Design review of the part built by this model. Coordinates are the model's own, in mm. Face numbers are marked on the shaded views. A direction names the side the tool comes from. Round coordinates to 2 decimals unless told otherwise and drop trailing zeros. Order: outer loops, then holes, each group sorted by start corner. A loop starts at its lowest first (then second) coordinate and runs counter-clockwise, first axis right, second up. Notation, with made-up numbers: (27.5, 29.25) - (59.5, 29.25) arc R20 cw to (59.5, 43.25) - close; hole circle Ø7 at (62, 16.5). An arc over 180 degrees is marked (long way). Write item = value, one per line.
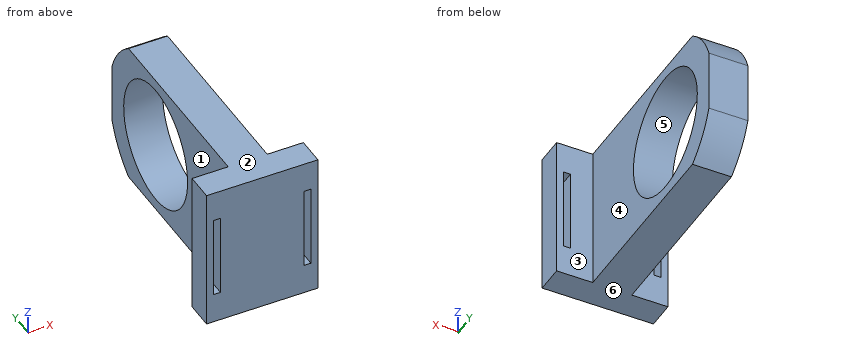
from build123d import *

# Parameters (mm, degrees)
SKETCH1_W           = 20
SKETCH1_H           = 26
SKETCH1_W_2         = 1.25
SKETCH1_H_2         = 15
BOSS_EXTRUDE5_DEPTH = 5
SKETCH3_W           = 7
SKETCH3_H           = 26
BOSS_EXTRUDE6_DEPTH = 40
CUT_EXTRUDE1_REACH  = 55.696
SKETCH5_R           = 11


with BuildPart() as part:
    # Sketch1 → Boss-Extrude5 (new body)
    with BuildSketch(Plane(origin=(0, 0, 0), x_dir=(1, 0, 0), z_dir=(0, 1, 0))):
        with Locations((10, 13)):
            Rectangle(SKETCH1_W, SKETCH1_H)
        with Locations((1.875, 13)):
            Rectangle(SKETCH1_W_2, SKETCH1_H_2, mode=Mode.SUBTRACT)
        with Locations((18.125784532, 13)):
            Rectangle(SKETCH1_W_2, SKETCH1_H_2, mode=Mode.SUBTRACT)
    extrude(amount=BOSS_EXTRUDE5_DEPTH)

    # Sketch3 → Boss-Extrude6 (add)
    with BuildSketch(Plane(origin=(0, 5, 0), x_dir=(1, 0, 0), z_dir=(0, 1, 0))):
        with Locations((10, 13)):
            Rectangle(SKETCH3_W, SKETCH3_H)
    extrude(amount=BOSS_EXTRUDE6_DEPTH)

    # Sketch5 → Cut-Extrude1 (cut, up to next)
    with BuildSketch(Plane(origin=(13.5, 0, 0), x_dir=(0, 0, -1), z_dir=(1, 0, 0)), mode=Mode.PRIVATE) as cut_extrude1_sk1:
        with Locations((13, 30)):
            Circle(SKETCH5_R)
    cut_extrude1_tool1 = extrude(cut_extrude1_sk1.sketch, amount=-CUT_EXTRUDE1_REACH, mode=Mode.PRIVATE) & part.part
    # Sketch5 → Cut-Extrude1 (cut, up to next)
    with BuildSketch(Plane(origin=(13.5, 0, 0), x_dir=(0, 0, -1), z_dir=(1, 0, 0)), mode=Mode.PRIVATE) as cut_extrude1_sk2:
        with BuildLine():
            Line((7.432235637, 45), (0, 45))
            Line((0, 45), (0, 39.327379053))
            ThreePointArc((0, 39.327379053), (3.292522189, 42.718682107), (7.432235637, 45))
        make_face()
    cut_extrude1_tool2 = extrude(cut_extrude1_sk2.sketch, amount=-CUT_EXTRUDE1_REACH, mode=Mode.PRIVATE) & part.part
    # Sketch5 → Cut-Extrude1 (cut, up to next)
    with BuildSketch(Plane(origin=(13.5, 0, 0), x_dir=(0, 0, -1), z_dir=(1, 0, 0)), mode=Mode.PRIVATE) as cut_extrude1_sk3:
        with BuildLine():
            Line((26, 39.327379053), (26, 45))
            Line((26, 45), (18.567764363, 45))
            ThreePointArc((18.567764363, 45), (22.707477811, 42.718682107), (26, 39.327379053))
        make_face()
    cut_extrude1_tool3 = extrude(cut_extrude1_sk3.sketch, amount=-CUT_EXTRUDE1_REACH, mode=Mode.PRIVATE) & part.part
    add(cut_extrude1_tool1.solids().sort_by_distance((13.5, 30, -13))[0], mode=Mode.SUBTRACT)
    add(cut_extrude1_tool2.solids().sort_by_distance((13.5, 43.298273, -2.197768))[0], mode=Mode.SUBTRACT)
    add(cut_extrude1_tool3.solids().sort_by_distance((13.5, 43.298273, -23.802232))[0], mode=Mode.SUBTRACT)


solid = part.part
1) We need section C-C on z = -13. Write out the cut boundary in (x, y), and give its area (4 significant figures).
Findings:
outline = (0, 0) - (1.25, 0) - (1.25, 5) - (0, 5) - close; (2.5, 0) - (17.5, 0) - (17.5, 5) - (13.5, 5) - (13.5, 19) - (6.5, 19) - (6.5, 5) - (2.5, 5) - close; (6.5, 41) - (13.5, 41) - (13.5, 45) - (6.5, 45) - close; (18.75, 0) - (20, 0) - (20, 5) - (18.75, 5) - close
area = 213.5 mm^2
2) To check wall thickness, follow L1, parallel to Y at x = 8, z = -13; L2, parallel to X at y = 39, z = -4; L3, parallel to Y at x = 17, z = -14.5. State the ranges of each line that lie inside material, in increasing order. Write a range as from..to.
Findings:
L1 = 0..19, 41..45
L2 = 6.5..13.5
L3 = 0..5
3) Clearance check with flat-ended pins moving along their axes: pin 1 Ø2 at (x, z) = (16.5, -13) entering from +Y; pin 2 Ø6 at (y, z) = (9, -5.5) entering from -X; pin 3 Ø2 at (x, y) = (15.5, 35.5) entering from -Z. State where each tip first meets the part, or that it passes through.
Findings:
pin_1 = 5
pin_2 = 6.5
pin_3 = through
4) For the marked faces 1, 2 and 3, list the 3-axis set-ups (+Z, -Z, +X, -X, +Y, -Y) from which the entire face can be reached by the end or side of a thin tool; tool diameter is ignored.
Findings:
face_1 = +Z, -Z, -X, +Y
face_2 = +Z, +X, -X, +Y, -Y
face_3 = +Z, -Z, +X, +Y
5) We need section B-B on y = 4.5. Write out the cut boundary in (x, z).
Findings:
outline = (0, -26) - (20, -26) - (20, 0) - (0, 0) - close; hole (1.25, -20.5) - (2.5, -20.5) - (2.5, -5.5) - (1.25, -5.5) - close; hole (17.5, -20.5) - (18.75, -20.5) - (18.75, -5.5) - (17.5, -5.5) - close
6) The part is to be moulded in two halves that separate along Z. For the marked faces 4, 5 and 6, say which applies: released by +Z, released by -Z, zero draft, split by the parting line, or undercut.
Findings:
face_4 = zero draft
face_5 = undercut
face_6 = released by -Z
7) We need section A-A on x = 18. Write out the cut boundary in (y, z).
Findings:
outline = (0, -26) - (5, -26) - (5, -20.5) - (0, -20.5) - close; (0, -5.5) - (5, -5.5) - (5, 0) - (0, 0) - close
8) We need section D-D on y = 30. Write out the cut boundary in (x, z), and give its area (3 significant figures).
Findings:
outline = (6.5, -26) - (13.5, -26) - (13.5, -24) - (6.5, -24) - close; (6.5, -2) - (13.5, -2) - (13.5, 0) - (6.5, 0) - close
area = 28.0 mm^2
